Read the model definition and answer for the solid it produces. Units are mm, in the model's axes. Round coordinates to 2 decimals unless told otherwise and drop trailing zeros. Order: outer loops, then holes, each group sorted by start corner. A loop starts at its lowest first (then second) coordinate and runs counter-clockwise, first axis right, second up. Notation, with made-up numbers: (-21.5, 46.5) - (28.5, 46.5) arc R17 cw to (28.5, 66.5) - close; hole circle Ø10 at (67, -22). An arc over 180 degrees is marked (long way). Answer as a JSON object with one key per item and string values. Group by question number.
Q1. A cutting plane is placed at A-A on y = -45. Determine the outline of the cut face in (x, z), and give its area (3 significant figures).
Q2. A cutting plane is placed at D-D on y = 26. Determine the outline of the cut face in (x, z).
Q3. Given pin 1 Ø2.5 at (x, y) = (-34.01, 0) entering from +Z; pin 2 Ø2 at (y, z) = (26.5, 4.5) entering from +X, each flat-ended and moving along its own axis, determine where each tip first touches the part or whether it passes through.
Q4. A cutting plane is placed at B-B on x = 17. Determine the outline of the cut face in (y, z), and give its area (3 significant figures).
Q5. A cutting plane is placed at C-C on z = 3.1. Count the separate pieces of the cut face and the enclosed holes in it, and give its area (3 significant figures).
Q6. Consider line 1 (Y direction, x = 0, z = 3.85); line 2 (Y direction, x = -8.5, z = 3.85); line 3 (X direction, y = 1, z = 2.7). Determine where each line is inside the solid, lowest interval first.
```python
from build123d import *

# Parameters (mm, degrees)
SKETCH1_R           = 37.5
SKETCH1_R_2         = 29.5
BOSS_EXTRUDE1_DEPTH = 5
SKETCH12_R          = 2
CUT_EXTRUDE8_DEPTH  = 7
SKETCH9_R           = 1.5
CUT_EXTRUDE5_DEPTH  = 7


with BuildPart() as part:
    # Sketch1 → Boss-Extrude1 (new body)
    # profile 1 of 2: a face of its own
    with BuildSketch(Plane.XY):
        Circle(SKETCH1_R)
        Circle(SKETCH1_R_2, mode=Mode.SUBTRACT)
    # profile 2 of 2: a face of its own
    with BuildSketch(Plane.XY):
        with BuildLine():
            Line((-15, -70), (15, -70))
            Line((15, -70), (35.350308448, -12.514219618))
            ThreePointArc((35.350308448, -12.514219618), (0, -37.5), (-35.350308448, -12.514219618))
            Line((-35.350308448, -12.514219618), (-15, -70))
        make_face()
    extrude(amount=BOSS_EXTRUDE1_DEPTH)

    # Sketch12 → Cut-Extrude8 (cut)
    with BuildSketch(Plane(origin=(0, 0, 0), x_dir=(-1, 0, 0), z_dir=(0, 0, -1))):
        with Locations((-12.5, -45)):
            Circle(SKETCH12_R)
        with Locations((12.5, -45)):
            Circle(SKETCH12_R)
        with Locations((-10, -60)):
            Circle(SKETCH12_R)
        with Locations((10, -60)):
            Circle(SKETCH12_R)
        with Locations((0, -45)):
            Circle(SKETCH12_R)
        with Locations((0, -60)):
            Circle(SKETCH12_R)
    extrude(amount=-CUT_EXTRUDE8_DEPTH, mode=Mode.SUBTRACT)

    # Sketch9 → Cut-Extrude5 (cut)
    with BuildSketch(Plane.XY.offset(5)):
        with Locations((17.005, 29.453523983)):
            Circle(SKETCH9_R)
        with Locations((34.01, 0)):
            Circle(SKETCH9_R)
        with Locations((17.005, -29.453523983)):
            Circle(SKETCH9_R)
        with Locations((-17.005, -29.453523983)):
            Circle(SKETCH9_R)
        with Locations((-34.01, 0)):
            Circle(SKETCH9_R)
        with Locations((-17.005, 29.453523983)):
            Circle(SKETCH9_R)
    extrude(amount=-CUT_EXTRUDE5_DEPTH, mode=Mode.SUBTRACT)


solid = part.part
```
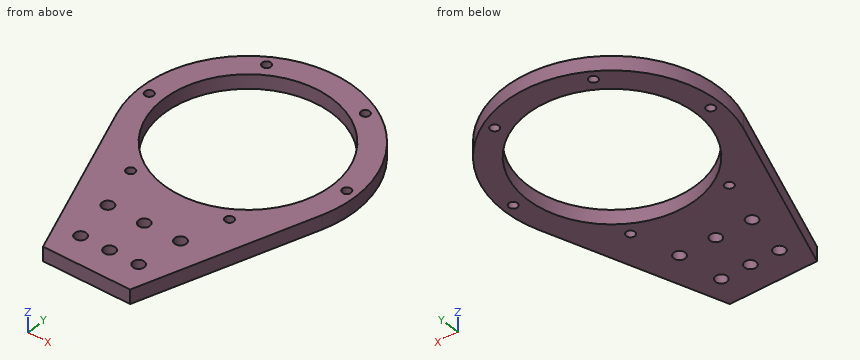
Result set:
{
 "1": {"outline": "(-23.85, 0) - (-14.5, 0) - (-14.5, 5) - (-23.85, 5) - close; (-10.5, 0) - (-2, 0) - (-2, 5) - (-10.5, 5) - close; (2, 0) - (10.5, 0) - (10.5, 5) - (2, 5) - close; (14.5, 0) - (23.85, 0) - (23.85, 5) - (14.5, 5) - close", "area": "179 mm²"},
 "2": {"outline": "(-27.02, 0) - (-13.94, 0) - (-13.94, 5) - (-27.02, 5) - close; (13.94, 0) - (27.02, 0) - (27.02, 5) - (13.94, 5) - close"},
 "3": {"pin 1": "passes through", "pin 2": "stops at x = 27.5"},
 "4": {"outline": "(-64.35, 0) - (-30.95, 0) - (-30.95, 5) - (-64.35, 5) - close; (-27.95, 0) - (-24.11, 0) - (-24.11, 5) - (-27.95, 5) - close; (24.11, 0) - (27.95, 0) - (27.95, 5) - (24.11, 5) - close; (30.95, 0) - (33.43, 0) - (33.43, 5) - (30.95, 5) - close", "area": "218 mm²"},
 "5": {"separate pieces": "1", "enclosed holes": "13", "area": "3,170 mm²"},
 "6": {"line 1": "y = -70 to -62, -58 to -47, -43 to -29.5, 29.5 to 37.5", "line 2": "y = -70 to -61.32, -58.68 to -28.25, 28.25 to 36.52", "line 3": "x = -37.49 to -35.13, -32.89 to -29.48, 29.48 to 32.89, 35.13 to 37.49"}
}
